Verification items for the finished model (mm, model axes). A direction names the side the tool comes from. Round coordinates to 2 decimals unless told otherwise and drop trailing zeros. Return JSON: item names as keys, results as strings. Group by question number.
1) Scan lines: L1, parallel to X at y = -1, z = 80; L2, parallel to X at y = -4, z = 200. Record each from-to range of solid material in increasing order.
2) Tool access check on faces 1 (the flat face through (3, -2, 280)), 2 (the cylindrical face through (3.588, -1.479, 168.002)). Record the directions out of +Z, -Z, +X, -X, +Y, -Y that give a thin tool (end or side, any length) a straight path to the whole face; none if there is none.
3) Draft check along X on faces 3 (the flat face through (3, -4.8, 167)), 4 (the flat face through (0, -2, 167)), 5 (the cylindrical face through (3.588, -1.479, 258.002)), 6 (the flat face through (2.6, -3, 185.9)). Enter one of: pulls with the +X half, pulls with the -X half, needs draft (parallel to the pull), parting line crosses it, or undercut.
4) Depth check by flat-ended pin: pin 1 (1.2 mm diameter, centred on x = 3.5, z = 140, fed in from +Y); pin 2 (2 mm diameter, centred on x = 4, z = 110, fed in from +Y); pin 3 (2.5 mm diameter, centred on x = 3.5, z = 215, fed in from -Y). Enter the tip coordinate at first touch or a pass-through.
5) Section check A-A on y = -1.75. State how many separate pieces and enclosed holes the cut face has, plus the area to 3 significant figures.
```python
from build123d import *

# Parameters (mm, degrees)
SKETCH_1_W             = 7
SKETCH_1_H             = 4.8
EXTRUDE_1_DEPTH        = 280
SKETCH_2_R             = 2
CUT_EXTRUDE_1_DEPTH    = 3
PATTERN_LINEAR_1_COUNT = 19
PATTERN_LINEAR_1_PITCH = 15
SKETCH_3_R             = 1
CUT_EXTRUDE_2_DEPTH    = 3
PATTERN_LINEAR_2_COUNT = 19
PATTERN_LINEAR_2_PITCH = 15
SKETCH_4_W             = 7
SKETCH_4_H             = 58
CUT_EXTRUDE_3_DEPTH    = 10


with BuildPart() as part:
    # 草图1 → 凸台-拉伸1 (new body)
    with BuildSketch(Plane.XY):
        with Locations((3.5, -2.4)):
            Rectangle(SKETCH_1_W, SKETCH_1_H)
    extrude(amount=EXTRUDE_1_DEPTH)

    # 草图2 → 切除-拉伸1 (cut)
    with BuildSketch(Plane(origin=(0, 0, 0), x_dir=(1, 0, 0), z_dir=(0, 1, 0))):
        with Locations(Location((3.5, -5, 0), (0, 0, 270))):
            Circle(SKETCH_2_R)
    cut_extrude_1 = extrude(amount=-CUT_EXTRUDE_1_DEPTH, mode=Mode.SUBTRACT)

    # 阵列(线性)1: 切除-拉伸1 ×19
    with Locations(*[(0, 0, i * PATTERN_LINEAR_1_PITCH) for i in range(1, PATTERN_LINEAR_1_COUNT)]):
        add(cut_extrude_1, mode=Mode.SUBTRACT)

    # 草图3 → 切除-拉伸2 (cut)
    with BuildSketch(Plane(origin=(0, -4.8, 0), x_dir=(-1, 0, 0), z_dir=(0, -1, 0))):
        with Locations(Location((-3.5, -5, 0), (0, 0, 90))):
            Circle(SKETCH_3_R)
    cut_extrude_2 = extrude(amount=-CUT_EXTRUDE_2_DEPTH, mode=Mode.SUBTRACT)

    # 阵列(线性)2: 切除-拉伸2 ×19
    with Locations(*[(0, 0, i * PATTERN_LINEAR_2_PITCH) for i in range(1, PATTERN_LINEAR_2_COUNT)]):
        add(cut_extrude_2, mode=Mode.SUBTRACT)

    # 草图4 → 切除-拉伸3 (cut)
    with BuildSketch(Plane(origin=(0, 0, 0), x_dir=(1, 0, 0), z_dir=(0, 1, 0))):
        with Locations((3.5, -29)):
            Rectangle(SKETCH_4_W, SKETCH_4_H)
    extrude(amount=-CUT_EXTRUDE_3_DEPTH, mode=Mode.SUBTRACT)


solid = part.part
```
Check result:
{
 "1": {"L1": "0 to 1.5, 5.5 to 7", "L2": "0 to 2.5, 4.5 to 7"},
 "2": {"face 1": "+Z, +X, -X, +Y, -Y", "face 2": "+Y"},
 "3": {"face 3": "needs draft", "face 4": "pulls with the -X half", "face 5": "undercut", "face 6": "undercut"},
 "4": {"pin 1": "through", "pin 2": "y = -3", "pin 3": "y = -4.8"},
 "5": {"separate pieces": "1", "enclosed holes": "15", "area": "1,370 mm^2"}
}
